```python
from build123d import *

# Parameters (mm, degrees)
F1_DEPTH = 12.7
F2_R     = 5.08


with BuildPart() as f1:
    # F0 (on Front) → F1 (new body)
    with BuildSketch(Plane.XZ):
        with BuildLine():
            Line((-28.5442825407, -19.2357096821), (-15.6568741476, -19.2357096821))
            ThreePointArc((-15.6568741476, -19.2357096821), (-54.678540264, -30.1371803507), (-15.6568741476, -41.0386510193))
            Line((-15.6568741476, -41.0386510193), (-28.5442825407, -41.0386510193))
            Line((-28.5442825407, -41.0386510193), (-28.5442825407, -19.2357096821))
        make_face()
        with BuildLine():
            Line((42.9155228194, -41.0386510193), (42.9155228194, -19.2357096821))
            Line((42.9155228194, -19.2357096821), (31.4341556288, -19.2357096821))
            ThreePointArc((31.4341556288, -19.2357096821), (28.3832827885, -30.1371803507), (31.4341556288, -41.0386510193))
            Line((31.4341556288, -41.0386510193), (42.9155228194, -41.0386510193))
        make_face()
        with BuildLine():
            ThreePointArc((31.4341556288, -41.0386510193), (28.3832827885, -30.1371803507), (31.4341556288, -19.2357096821))
            Line((31.4341556288, -19.2357096821), (-15.6568741476, -19.2357096821))
            ThreePointArc((-15.6568741476, -19.2357096821), (-13.3870219255, -24.4777329529), (-12.6113336936, -30.1371803507))
            ThreePointArc((-12.6113336936, -30.1371803507), (-13.3870219255, -35.7966277486), (-15.6568741476, -41.0386510193))
            Line((-15.6568741476, -41.0386510193), (31.4341556288, -41.0386510193))
        make_face()
        with BuildLine():
            ThreePointArc((-12.6113336936, -30.1371803507), (-13.3870219255, -24.4777329529), (-15.6568741476, -19.2357096821))
            Line((-15.6568741476, -19.2357096821), (-28.5442825407, -19.2357096821))
            Line((-28.5442825407, -19.2357096821), (-28.5442825407, -41.0386510193))
            Line((-28.5442825407, -41.0386510193), (-15.6568741476, -41.0386510193))
            ThreePointArc((-15.6568741476, -41.0386510193), (-13.3870219255, -35.7966277486), (-12.6113336936, -30.1371803507))
        make_face()
        with BuildLine():
            Line((31.4341556288, -19.2357096821), (42.9155228194, -19.2357096821))
            Line((42.9155228194, -19.2357096821), (42.9155228194, -41.0386510193))
            Line((42.9155228194, -41.0386510193), (31.4341556288, -41.0386510193))
            ThreePointArc((31.4341556288, -41.0386510193), (55.0456161452, -50.3622536115), (70.3876187723, -30.1371803507))
            ThreePointArc((70.3876187723, -30.1371803507), (55.0456161452, -9.91210709), (31.4341556288, -19.2357096821))
        make_face()
    extrude(amount=F1_DEPTH)

    # F2
    f2_edges = [f1.edges().sort_by_distance(p)[0] for p in [
        (-54.67854, 0, -30.13718),
        (-15.656874, -6.35, -19.23571),
        (-15.656874, -6.35, -41.038651),
        (-54.67854, -12.7, -30.13718),
        (7.888641, 0, -41.038651),
        (70.387619, 0, -30.13718),
        (7.888641, 0, -19.23571),
        (31.434156, -6.35, -41.038651),
        (31.434156, -6.35, -19.23571),
        (70.387619, -12.7, -30.13718),
        (7.888641, -12.7, -41.038651),
        (7.888641, -12.7, -19.23571),
    ]]
    fillet(f2_edges, radius=F2_R)


solid = f1.part
```
The listing builds one solid part. Answer for the finished solid, in the listing's coordinates (mm). A direction names the side the tool comes from. Give positions to 0.01 mm unless a question says otherwise; leave off trailing zeros. Write each loop counter-clockwise with the first axis right and the second up, starting at its lowest first coordinate (ties: lowest second). Pieces come first, ordered by that corner, then holes. Notation, with made-up numbers: (-8.5, 7) -> (7.5, 7) arc R18 cw to (7.5, 23) -> close; hole circle Ø11 at (28.25, 32). An arc over 180 degrees is marked (long way). Write item = value, one per line. Start each with the question number.
1) The part is cut by section A-A, the plane x = 5. Determine the outline of the cut face in (y, z), and give its area (3 significant figures).
2) Each of these flat-tipped pins is pushed along its axis until it touches: pin 1 (4 mm diameter, centred on x = 38, y = -11, fed in from -Z); pin 2 (1.5 mm diameter, centred on y = -4, z = -34, fed in from -X); pin 3 (4 mm diameter, centred on y = -3, z = -28.5, fed in from -X). Where does it stop, or does it pass through?
3) Straight lines are drawn through the part: line 1 along Z through (x, y) = (5.5, -5.5); line 2 along X through (y, z) = (-8, -30); line 3 along Z through (x, y) = (49.5, -5). For each, find the intervals that lie inside material, in ascending order.
4) Which of the six approach directions +Z, -Z, +X, -X, +Y, -Y give full straight-line access (tool end or side, diameter ignored) to faces 5 (the face through (8.18, -11.17, -39.59)), 6 (the face through (8, -2, -40)), 7 (the face through (8, -6, -41.039)), 8 (the face through (-15.26, -6.37, -18.7)), 9 (the face through (7.6, -11.17, -20.68))?
5) The part is cut by section B-B, the plane y = -3. Determine the outline of the cut face in (x, z).
6) Determine the mould class of faces 1 (the face through (-54.666, -6.332, -29.406)), 2 (the face through (-15.259, -6.368, -41.572)), 3 (the face through (7, 0, -30)), 4 (the face through (8, -6, -19.236)) for opening direction Z: +Z half, -Z half, draft (parallel to the pull), parting line (faces both ways), or undercut.
Solutions:
q1.outline = (-12.7, -35.96) arc R5.08 ccw to (-7.62, -41.04) -> (-5.08, -41.04) arc R5.08 ccw to (0, -35.96) -> (0, -24.32) arc R5.08 ccw to (-5.08, -19.24) -> (-7.62, -19.24) arc R5.08 ccw to (-12.7, -24.32) -> close
q1.area = 255 mm²
q2.pin_1 = -48.17
q2.pin_2 = -54.38
q2.pin_3 = -54.66
q3.line_1 = -41.04 to -19.24
q3.line_2 = -54.66 to 70.37
q3.line_3 = -51.14 to -9.14
q4.face_5 = -Z, -Y
q4.face_6 = -Z, +Y
q4.face_7 = -Z, +Y, -Y
q4.face_8 = +Z, +Y, -Y
q4.face_9 = +Z, -Y
q5.outline = (-17.36, -42.74) arc R5.53 cw to (-12.99, -40.59) -> (28.77, -40.59) arc R5.53 cw to (33.14, -42.73) arc R20.56 ccw (long way) to (33.14, -17.54) arc R5.53 cw to (28.77, -19.68) -> (-12.99, -19.68) arc R5.53 cw to (-17.36, -17.54) arc R20.59 ccw (long way) to start
q6.face_1 = parting line
q6.face_2 = -Z half
q6.face_3 = draft
q6.face_4 = +Z half
